```python
from build123d import *

# Parameters (mm, degrees)
F0_R     = 2
F1_DEPTH = 3


with BuildPart() as f1:
    # F0 (on Top) → F1 (new body)
    with BuildSketch(Plane.XY):
        with BuildLine():
            ThreePointArc((68, 9), (67.12132, 11.12132), (65, 12))
            Line((65, 12), (-9, 12))
            ThreePointArc((-9, 12), (-11.12132, 11.12132), (-12, 9))
            Line((-12, 9), (-12, -5))
            ThreePointArc((-12, -5), (-11.12132, -7.12132), (-9, -8))
            Line((-9, -8), (65, -8))
            ThreePointArc((65, -8), (67.12132, -7.12132), (68, -5))
            Line((68, -5), (68, 9))
        make_face()
        Circle(F0_R, mode=Mode.SUBTRACT)
        with Locations((20, 0)):
            Circle(F0_R, mode=Mode.SUBTRACT)
        with Locations((40, 0)):
            Circle(F0_R, mode=Mode.SUBTRACT)
        with Locations((60, 0)):
            Circle(F0_R, mode=Mode.SUBTRACT)
    extrude(amount=F1_DEPTH)


solid = f1.part
```
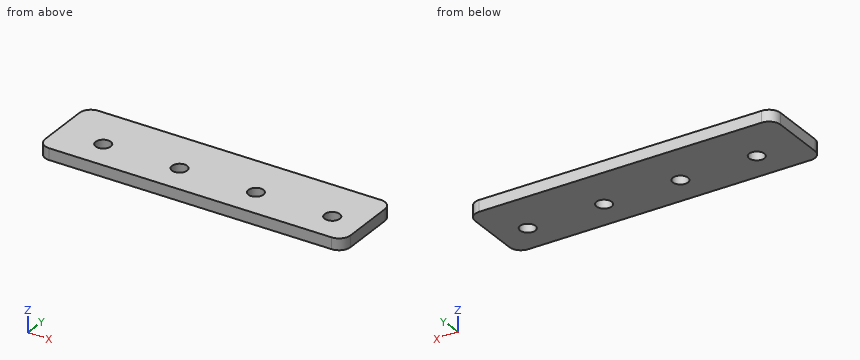
Verification items for the finished model (mm, model axes). Coordinates: 2 decimals unless noted, no trailing zeros. Write each loop counter-clockwise with the first axis right and the second up, starting at its lowest first coordinate (ties: lowest second). Pieces come first, ordered by that corner, then holes. Notation, with made-up numbers: (-24, 13.25) - (3, 13.25) arc R22 ccw to (3, 27.25) - close; hole circle Ø3 at (-11, -7.5). An arc over 180 degrees is marked (long way). Write item = value, one per line.
Q1. Material ranges on L1, parallel to Y at x = 20, z = 0.75; L2, parallel to X at y = 1.5, z = 0.65; L3, parallel to X at y = 1.25, z = 0.45, recorded low to high. Write a range as from..to.
Answer:
L1 = -8..-2, 2..12
L2 = -12..-1.32, 1.32..18.68, 21.32..38.68, 41.32..58.68, 61.32..68
L3 = -12..-1.56, 1.56..18.44, 21.56..38.44, 41.56..58.44, 61.56..68
Q2. Cross-section at D-D (y = -7). Enter the section's corners in (x, z), plus the area to 3 significant figures.
Answer:
outline = (-11.24, 0) - (67.24, 0) - (67.24, 3) - (-11.24, 3) - close
area = 235 mm²
Q3. Cross-section at A-A (y = 0). Enter the section's corners in (x, z).
Answer:
outline = (-12, 0) - (-2, 0) - (-2, 3) - (-12, 3) - close; (2, 0) - (18, 0) - (18, 3) - (2, 3) - close; (22, 0) - (38, 0) - (38, 3) - (22, 3) - close; (42, 0) - (58, 0) - (58, 3) - (42, 3) - close; (62, 0) - (68, 0) - (68, 3) - (62, 3) - close
Q4. Cross-section at B-B (x = 20). Enter the section's corners in (y, z), plus the area to 3 significant figures.
Answer:
outline = (-8, 0) - (-2, 0) - (-2, 3) - (-8, 3) - close; (2, 0) - (12, 0) - (12, 3) - (2, 3) - close
area = 48.0 mm²
Q5. Cross-section at C-C (z = 2.25). Enter the section's corners in (x, y), plus the area to 3 significant figures.
Answer:
outline = (-12, -5) arc R3 ccw to (-9, -8) - (65, -8) arc R3 ccw to (68, -5) - (68, 9) arc R3 ccw to (65, 12) - (-9, 12) arc R3 ccw to (-12, 9) - close; hole circle Ø4 at (0, 0); hole circle Ø4 at (20, 0); hole circle Ø4 at (40, 0); hole circle Ø4 at (60, 0)
area = 1,540 mm²
